```python
from build123d import *

# Parameters (mm, degrees)
SKETCH1_W            = 560
SKETCH1_H            = 410
BOSS_EXTRUDE1_DEPTH  = 3
SKETCH2_R            = 9.9
BOSS_EXTRUDE2_DEPTH  = 3
SKETCH3_W            = 30
SKETCH3_H            = 20
BOSS_EXTRUDE3_DEPTH  = 92
LPATTERN1_COUNT      = 2
LPATTERN1_PITCH      = 210
BOSS_EXTRUDE4_REACH  = 654.324
SKETCH4_W            = 15
SKETCH4_H            = 15
FILLET1_R            = 10
FILLET1_OF_MIRROR1_R = 10
SKETCH5_R            = 2.65
CUT_EXTRUDE1_DEPTH   = 92
CUT_EXTRUDE2_DEPTH   = 653.32449747


with BuildPart() as part:
    # Sketch1 → Boss-Extrude1 (new body)
    with BuildSketch(Plane(origin=(0, 0, 0), x_dir=(1, 0, 0), z_dir=(0, 1, 0))):
        with Locations((250, 185)):
            Rectangle(SKETCH1_W, SKETCH1_H)
        with BuildLine():
            Line((500, 130), (500, 40))
            Line((500, 40), (475, 40))
            ThreePointArc((475, 40), (464.393398282, 35.606601718), (460, 25))
            Line((460, 25), (460, 15))
            ThreePointArc((460, 15), (464.393398282, 4.393398282), (475, 0))
            Line((475, 0), (25, 0))
            ThreePointArc((25, 0), (35.606601718, 4.393398282), (40, 15))
            Line((40, 15), (40, 25))
            ThreePointArc((40, 25), (35.606601718, 35.606601718), (25, 40))
            Line((25, 40), (0, 40))
            Line((0, 40), (0, 130))
            Line((0, 130), (25, 130))
            ThreePointArc((25, 130), (35.606601718, 134.393398282), (40, 145))
            Line((40, 145), (40, 225))
            ThreePointArc((40, 225), (35.606601718, 235.606601718), (25, 240))
            Line((25, 240), (0, 240))
            Line((0, 240), (0, 330))
            Line((0, 330), (25, 330))
            ThreePointArc((25, 330), (35.606601718, 334.393398282), (40, 345))
            Line((40, 345), (40, 355))
            ThreePointArc((40, 355), (35.606601718, 365.606601718), (25, 370))
            Line((25, 370), (475, 370))
            ThreePointArc((475, 370), (464.393398282, 365.606601718), (460, 355))
            Line((460, 355), (460, 345))
            ThreePointArc((460, 345), (464.393398282, 334.393398282), (475, 330))
            Line((475, 330), (500, 330))
            Line((500, 330), (500, 240))
            Line((500, 240), (475, 240))
            ThreePointArc((475, 240), (464.393398282, 235.606601718), (460, 225))
            Line((460, 225), (460, 145))
            ThreePointArc((460, 145), (464.393398282, 134.393398282), (475, 130))
            Line((475, 130), (500, 130))
        make_face(mode=Mode.SUBTRACT)
    extrude(amount=BOSS_EXTRUDE1_DEPTH)

    # Sketch2 → Boss-Extrude2 (add)
    with BuildSketch(Plane(origin=(0, 3, 0), x_dir=(1, 0, 0), z_dir=(0, 1, 0))):
        with Locations(Location((20, 150, 0), (0, 0, 270))):
            Circle(SKETCH2_R)
        with Locations(Location((20, 220, 0), (0, 0, 270))):
            Circle(SKETCH2_R)
        with Locations(Location((20, 350, 0), (0, 0, 270))):
            Circle(SKETCH2_R)
        with Locations(Location((20, 20, 0), (0, 0, 270))):
            Circle(SKETCH2_R)
        with Locations(Location((480, 150, 0), (0, 0, 270))):
            Circle(SKETCH2_R)
        with Locations(Location((480, 220, 0), (0, 0, 270))):
            Circle(SKETCH2_R)
        with Locations(Location((480, 350, 0), (0, 0, 270))):
            Circle(SKETCH2_R)
        with Locations(Location((480, 20, 0), (0, 0, 270))):
            Circle(SKETCH2_R)
    extrude(amount=BOSS_EXTRUDE2_DEPTH)

    # Sketch3 → Boss-Extrude3 (add)
    with BuildSketch(Plane(origin=(0, 3, 0), x_dir=(1, 0, 0), z_dir=(0, 1, 0))):
        with Locations((545, 287.5)):
            Rectangle(SKETCH3_W, SKETCH3_H)
        with Locations((-45, 287.5)):
            Rectangle(SKETCH3_W, SKETCH3_H)
    boss_extrude3 = extrude(amount=-BOSS_EXTRUDE3_DEPTH)

    # LPattern1: Boss-Extrude3 ×2
    with Locations(*[(0, 0, i * LPATTERN1_PITCH) for i in range(1, LPATTERN1_COUNT)]):
        add(boss_extrude3)

    # Boss-Extrude4: up to this face of the body (flat: up to its plane)
    boss_extrude4_end = Plane(part.part.faces().sort_by_distance((-45, -43, -297.5))[0])
    # Sketch4 → Boss-Extrude4 (add, up to the picked face)
    with BuildSketch(Plane.XY.offset(-67.5), mode=Mode.PRIVATE) as boss_extrude4_sk1:
        with Locations((522.5, -7.5)):
            Rectangle(SKETCH4_W, SKETCH4_H)
    boss_extrude4_tool1 = split(extrude(boss_extrude4_sk1.sketch, amount=-BOSS_EXTRUDE4_REACH, mode=Mode.PRIVATE), bisect_by=boss_extrude4_end, keep=Keep.BOTH, mode=Mode.PRIVATE)
    boss_extrude4 = boss_extrude4_tool1.solids().sort_by(Axis((522.5, -7.5, -67.5), (0, 0, -1)))[0]
    add(boss_extrude4)

    # Fillet1
    fillet1_edges = [part.edges().sort_by_distance(p)[0] for p in [
        (515, -15, -182.5),
    ]]
    fillet(fillet1_edges, radius=FILLET1_R)

    # Mirror1: Boss-Extrude4 across plane
    add(boss_extrude4.mirror(Plane(origin=(250, 0, 0), x_dir=(0, 0, 1), z_dir=(1, 0, 0))))

    # Fillet1 of Mirror1
    fillet1_of_mirror1_edges = [part.edges().sort_by_distance(p)[0] for p in [
        (-15, -15, -182.5),
    ]]
    fillet(fillet1_of_mirror1_edges, radius=FILLET1_OF_MIRROR1_R)

    # Sketch5 → Cut-Extrude1 (cut)
    with BuildSketch(Plane(origin=(-30, 0, 0), x_dir=(0, 0, -1), z_dir=(1, 0, 0))):
        with Locations((77.5, -79)):
            Circle(SKETCH5_R)
        with Locations((287.5, -79)):
            Circle(SKETCH5_R)
    cut_extrude1 = extrude(amount=-CUT_EXTRUDE1_DEPTH, mode=Mode.SUBTRACT)

    # Mirror2: Cut-Extrude1 across plane
    add(cut_extrude1.mirror(Plane(origin=(250, 0, 0), x_dir=(0, 0, 1), z_dir=(1, 0, 0))), mode=Mode.SUBTRACT)

    # Sketch6 → Cut-Extrude2 (cut, through all)
    with BuildSketch(Plane.XY.offset(-67.5)):
        Polygon((-45, -89), (-45, -30), (-30, -15), (-30, -89), align=None)
    cut_extrude2 = extrude(amount=-CUT_EXTRUDE2_DEPTH, mode=Mode.SUBTRACT)

    # Mirror3: Cut-Extrude2 across plane
    add(cut_extrude2.mirror(Plane(origin=(250, 0, 0), x_dir=(0, 0, 1), z_dir=(1, 0, 0))), mode=Mode.SUBTRACT)


solid = part.part
```
Geometry check sheet. Reference: the model listing, model coordinates, mm. A direction names the side the tool comes from. Round coordinates to 2 decimals unless told otherwise and drop trailing zeros. Loops run counter-clockwise (first coordinate to the right, second up) from the corner with the lowest first, then second, coordinate; pieces in that order, holes last. Notation, with made-up numbers: M 60.5,16.5 L 107.5,16.5 A20 ccw 107.5,39.5 Z; hole C 32.25,69 d7. An arc over 180 degrees is marked long. Return JSON: item names as keys, results as strings. Group by question number.
(1) Go/stop test with flat-tipped pins: pin 1 (9 mm diameter, centred on y = -5, z = -160, fed in from -X); pin 2 (0.9 mm diameter, centred on y = 2, z = -268, fed in from +X). Record where each tip stops, or that it passes through.
(2) Mould release check, pull along X, two halves, no side actions. Record for faces 5 (the face through (-53, -89, -78)), 6 (the face through (-60, -42, -77)), 7 (the face through (545, -60, -77)): pulls with the +X half, pulls with the -X half, needs draft (parallel to the pull), parting line crosses it, or undercut.
(3) Section check B-B, the plane x = 265. Enter the section's corners in (y, z).
(4) Scan lines: line 1 along Z through (x, y) = (550, -79); line 2 along X through (y, z) = (-41.5, -75); line 3 along X through (y, z) = (-2.5, -138). Record each from-to range of solid material in increasing order. Write a range as [from, to].
(5) Section check A-A, the plane y = -54. Enter the section's corners in (x, z), and give its area (3 significant figures).
(6) Set-up check for faces 1 (the face through (20, 6, -350)), 2 (the face through (545, -60, -287)), 3 (the face through (29.816, 4.479, -221.289)), 4 (the face through (464.51, 1.48, -235.72)): record each of +Z, -Z, +X, -X, +Y, -Y from which the full face is reachable in a straight line by a thin tool's end or side.
(7) Section check C-C, the plane z = -203.5. Enter the section's corners in (x, y).
(8) Section check D-D, the plane y = -24. Enter the section's corners in (x, z), and give its area (3 significant figures).
Data:
{
 "1": {"pin 1": "x = -30", "pin 2": "x = 530"},
 "2": {"face 5": "needs draft", "face 6": "pulls with the -X half", "face 7": "undercut"},
 "3": {"outline": "M 0,-390 L 3,-390 L 3,-370 L 0,-370 Z; M 0,0 L 3,0 L 3,20 L 0,20 Z"},
 "4": {"line 1": "[-297.5, -290.15], [-284.85, -277.5], [-87.5, -80.15], [-74.85, -67.5]", "line 2": "[-60, -45], [545, 560]", "line 3": "[-30, -15], [515, 530]"},
 "5": {"outline": "M -60,-297.5 L -45,-297.5 L -45,-277.5 L -60,-277.5 Z; M -60,-87.5 L -45,-87.5 L -45,-67.5 L -60,-67.5 Z; M 545,-297.5 L 560,-297.5 L 560,-277.5 L 545,-277.5 Z; M 545,-87.5 L 560,-87.5 L 560,-67.5 L 545,-67.5 Z", "area": "1,200 mm²"},
 "6": {"face 1": "+Z, -Z, +X, -X, +Y", "face 2": "+Z, -Z, -Y", "face 3": "+Y", "face 4": "+Y, -Y"},
 "7": {"outline": "M -30,-15 L -25,-15 A10 ccw -15,-5 L -15,0 L 40,0 L 40,3 L -30,3 Z; M 460,0 L 515,0 L 515,-5 A10 ccw 525,-15 L 530,-15 L 530,3 L 460,3 Z"},
 "8": {"outline": "M -60,-297.5 L -39,-297.5 L -39,-277.5 L -60,-277.5 Z; M -60,-87.5 L -39,-87.5 L -39,-67.5 L -60,-67.5 Z; M 539,-297.5 L 560,-297.5 L 560,-277.5 L 539,-277.5 Z; M 539,-87.5 L 560,-87.5 L 560,-67.5 L 539,-67.5 Z", "area": "1,680 mm²"}
}
